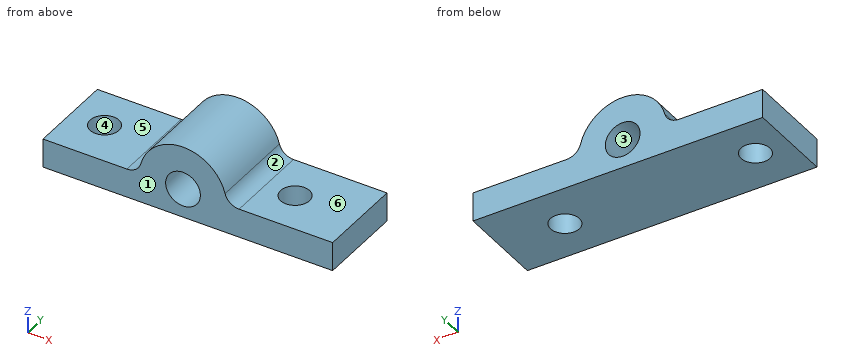
```python
from build123d import *

# Parameters (mm, degrees)
F0_R     = 7.62
F1_DEPTH = 38.1
F2_R     = 6.35
F3_DEPTH = 25.4


with BuildPart() as f1:
    # F0 (on Front) → F1 (new body)
    with BuildSketch(Plane.XZ):
        with BuildLine():
            Line((-64.016195, -28.264835), (62.983805, -28.264835))
            Line((62.983805, -28.264835), (62.983805, -15.564835))
            Line((62.983805, -15.564835), (21.960583, -15.564835))
            ThreePointArc((21.960583, -15.564835), (18.072018, -14.23495), (15.812222, -10.802335))
            ThreePointArc((15.812222, -10.802335), (-2.632861, 3.485165), (-21.077944, -10.802335))
            ThreePointArc((-21.077944, -10.802335), (-23.33774, -14.23495), (-27.226305, -15.564835))
            Line((-27.226305, -15.564835), (-64.016195, -15.564835))
            Line((-64.016195, -15.564835), (-64.016195, -28.264835))
        make_face()
        with Locations((-2.632861, -15.564835)):
            Circle(F0_R, mode=Mode.SUBTRACT)
    extrude(amount=F1_DEPTH)

    # F2 (on face) → F3 (cut)
    with BuildSketch(Plane.XY.offset(-15.564835)):
        with Locations((-49.384239, -18.341588)):
            Circle(F2_R)
        with Locations((34.943767, -19.611587)):
            Circle(F2_R)
    extrude(amount=-F3_DEPTH, mode=Mode.SUBTRACT)


solid = f1.part
```
CAD build for the part. Positions are in the model's coordinates, mm. Face numbers are marked on the shaded views. A direction names the side the tool comes from. Give positions to 0.01 mm unless a question says otherwise; leave off trailing zeros. Order: outer loops, then holes, each group sorted by start corner. A loop starts at its lowest first (then second) coordinate and runs counter-clockwise, first axis right, second up. Notation, with made-up numbers: M 71.25,-35 L 113.25,-35 A18 ccw 113.25,-14 Z; hole C 7.25,1 d6. An arc over 180 degrees is marked long. Put each result on its own line as item: value. Start each with the question number.
(1) Mould opens along Z. For the marked faces 1, 2 and 3 say: +Z half, -Z half, draft (parallel to the pull), parting line (faces both ways), or undercut.
(2) Drill centre lines: line 1 along X through (y, z) = (-19.5, -17); line 2 along X through (y, z) = (-18, -25); line 3 along X through (y, z) = (-32.5, -8.5). Where is each one in solid material? Low to high.
(3) Which spindle directions (+Z, -Z, +X, -X, +Y, -Y) get a long thin tool onto all of the face, cutting with end or side? Do the marked faces 4, 5 and 6. Say none if no direction does.
(4) Saw through at C-C, the plane x = -3. Write the cut outline in (y, z).
(5) Flat gauge pins, fed straight in: pin 1 Ø5 at (x, y) = (26.5, -14) entering from +Z; pin 2 Ø1.5 at (y, z) = (-11.5, -8) entering from -X; pin 3 Ø2 at (y, z) = (-19, -10.5) entering from +X. Where does each tip first touch, or does it go through?
(6) Saw through at D-D, the plane z = -9.5. Write the cut outline in (x, y).
(7) Saw through at B-B, the plane y = -16. Write the cut outline in (x, z).
(8) Saw through at A-A, the plane z = -20. Write the cut outline in (x, y), then the cut area to 3 significant figures.
Check result:
1. face 1: draft
1. face 2: +Z half
1. face 3: undercut
2. line 1: x = -64.02 to -55.63, -43.14 to -10.12, 4.85 to 28.59, 41.29 to 62.98
2. line 2: x = -64.02 to -55.73, -43.04 to 28.8, 41.09 to 62.98
2. line 3: x = -20.32 to -5.49, 0.22 to 15.06
3. face 4: +Z, -Z
3. face 5: +Z, -X, +Y, -Y
3. face 6: +Z, +X, +Y, -Y
4. outline: M -38.1,-28.26 L 0,-28.26 L 0,-23.18 L -38.1,-23.18 Z; M -38.1,-7.95 L 0,-7.95 L 0,3.48 L -38.1,3.48 Z
5. pin 1: stops at z = -15.56
5. pin 2: stops at x = -20.42
5. pin 3: stops at x = 16.04
6. outline: M -20.69,-38.1 L -7.25,-38.1 L -7.25,0 L -20.69,0 Z; M 1.98,-38.1 L 15.43,-38.1 L 15.43,0 L 1.98,0 Z
7. outline: M -64.02,-28.26 L -55.29,-28.26 L -55.29,-15.56 L -64.02,-15.56 Z; M -43.48,-28.26 L 29.72,-28.26 L 29.72,-15.56 L 21.96,-15.56 A6.35 cw 15.81,-10.8 A19.05 ccw -21.08,-10.8 A6.35 cw -27.23,-15.56 L -43.48,-15.56 Z; M 40.17,-28.26 L 62.98,-28.26 L 62.98,-15.56 L 40.17,-15.56 Z; hole C -2.63,-15.56 d15.24
8. outline: M -64.02,-38.1 L -8.83,-38.1 L -8.83,0 L -64.02,0 Z; M 3.56,-38.1 L 62.98,-38.1 L 62.98,0 L 3.56,0 Z; hole C -49.38,-18.34 d12.7; hole C 34.94,-19.61 d12.7
8. area: 4,110 mm2
